from build123d import *

# Parameters (mm, degrees)
F0_W     = 393.7
F0_H     = 165.1
F1_DEPTH = 19.05
F3_DEPTH = 558.8
F4_W     = 307.975
F4_H     = 533.4
F5_DEPTH = 88.9
F6_W     = 307.975
F6_H     = 533.4
F7_DEPTH = 6.35


with BuildPart() as f1:
    # F0 (on Front) → F1 (new body)
    with BuildSketch(Plane.XZ):
        Rectangle(F0_W, F0_H)
    extrude(amount=F1_DEPTH)

    # F2 (on face) → F3 (join)
    with BuildSketch(Plane(origin=(0, 0, 0), x_dir=(-1, 0, 0), z_dir=(0, 1, 0))):
        Polygon((-166.6875, -69.85), (0, -69.85), (166.6875, -69.85), (166.6875, 31.75), (-166.6875, 31.75), align=None)
    extrude(amount=F3_DEPTH)

    # F4 (on face) → F5 (cut)
    with BuildSketch(Plane.XY.offset(31.75)):
        with Locations((0, 279.4)):
            Rectangle(F4_W, F4_H)
    extrude(amount=-F5_DEPTH, mode=Mode.SUBTRACT)

    # F6 (on face) → F7 (cut)
    with BuildSketch(Plane(origin=(0, 0, -69.85), x_dir=(1, 0, 0), z_dir=(0, 0, -1))):
        with Locations((0, -279.4)):
            Rectangle(F6_W, F6_H)
    extrude(amount=-F7_DEPTH, mode=Mode.SUBTRACT)


solid = f1.part
Geometry check sheet. Reference: the model listing, model coordinates, mm. A direction names the side the tool comes from. Round coordinates to 2 decimals unless told otherwise and drop trailing zeros. Order: outer loops, then holes, each group sorted by start corner. A loop starts at its lowest first (then second) coordinate and runs counter-clockwise, first axis right, second up. Notation, with made-up numbers: (50, 60) -> (86, 60) arc R16 ccw to (86, 84) -> close; hole circle Ø4 at (41, 85.5). An arc over 180 degrees is marked (long way). Use one line per item in the form item = value.
1. Cross-section at C-C, the plane x = 144.5. Enter the section's corners in (y, z).
Working result:
outline = (-19.05, -82.55) -> (0, -82.55) -> (0, -69.85) -> (12.7, -69.85) -> (12.7, -63.5) -> (546.1, -63.5) -> (546.1, -69.85) -> (558.8, -69.85) -> (558.8, 31.75) -> (546.1, 31.75) -> (546.1, -57.15) -> (12.7, -57.15) -> (12.7, 31.75) -> (0, 31.75) -> (0, 82.55) -> (-19.05, 82.55) -> close
2. Cross-section at D-D, the plane z = 55. Enter the section's corners in (x, y).
Working result:
outline = (-196.85, -19.05) -> (196.85, -19.05) -> (196.85, 0) -> (-196.85, 0) -> close
3. Cross-section at A-A, the plane z = -13.5. Enter the section's corners in (x, y), plus the area to 3 significant figures.
Working result:
outline = (-196.85, -19.05) -> (196.85, -19.05) -> (196.85, 0) -> (166.69, 0) -> (166.69, 558.8) -> (-166.69, 558.8) -> (-166.69, 0) -> (-196.85, 0) -> close; hole (-153.99, 12.7) -> (153.99, 12.7) -> (153.99, 546.1) -> (-153.99, 546.1) -> close
area = 29,500 mm^2
4. Go/stop test with flat-tipped pins: pin 1 (3 mm diameter, centred on y = 317, z = -66.5, fed in from +X); pin 2 (1 mm diameter, centred on x = -70.5, y = 486.5, fed in from -Z); pin 3 (5 mm diameter, centred on y = 255.5, z = -66, fed in from -X). Record where each tip stops, or that it passes through.
Working result:
pin_1 = 166.69
pin_2 = -63.5
pin_3 = -166.69
5. Set-up check for faces 1 (the face through (161, 278, -69.85)), 2 (the face through (-2, 283, -57.15)), 3 (the face through (-161, 278, 31.75)), 4 (the face through (166.688, 275, -18)), 5 (the face through (-166.688, 275, -20)): record each of +Z, -Z, +X, -X, +Y, -Y from which the full face is reachable in a straight line by a thin tool's end or side.
Working result:
face_1 = -Z, +X, -X, +Y
face_2 = +Z
face_3 = +Z, +X, -X, +Y
face_4 = +Z, -Z, +X, +Y
face_5 = +Z, -Z, -X, +Y
6. Scan lines: line 1 along Y through (x, z) = (1, -56.5); line 2 along X through (y, z) = (482, 28.5); line 3 along Z through (x, y) = (-52, 427). Record each from-to range of solid material in increasing order. Write a range as from..to.
Working result:
line_1 = -19.05..12.7, 546.1..558.8
line_2 = -166.69..-153.99, 153.99..166.69
line_3 = -63.5..-57.15
7. Cross-section at B-B, the plane y = 298. Enter the section's corners in (x, z), plus the area to 3 significant figures.
Working result:
outline = (-166.69, -69.85) -> (-153.99, -69.85) -> (-153.99, -63.5) -> (153.99, -63.5) -> (153.99, -69.85) -> (166.69, -69.85) -> (166.69, 31.75) -> (153.99, 31.75) -> (153.99, -57.15) -> (-153.99, -57.15) -> (-153.99, 31.75) -> (-166.69, 31.75) -> close
area = 4,540 mm^2
8. Mould release check, pull along X, two halves, no side actions. Record for faces 6 (the face through (-196.85, -9, -1)), 7 (the face through (-2, 546.1, -12)), 8 (the face through (-3, -9, 82.55)): pulls with the +X half, pulls with the -X half, needs draft (parallel to the pull), parting line crosses it, or undercut.
Working result:
face_6 = pulls with the -X half
face_7 = undercut
face_8 = needs draft
